Input: part model. Units: mm. Frame: model coordinates. Face numbers are marked on the shaded views. A direction names the side the tool comes from. Round coordinates to 2 decimals unless told otherwise and drop trailing zeros. Loops run counter-clockwise (first coordinate to the right, second up) from the corner with the lowest first, then second, coordinate; pieces in that order, holes last. Notation, with made-up numbers: M 20.25,-35 L 40.25,-35 A16 cw 40.25,-20 Z; hole C -10.5,-14 d11. An arc over 180 degrees is marked long. Use one line per item in the form item = value. Start each with the question number.
Q1. Ray query, line 1 along Y through (x, z) = (45, 43); line 2 along X through (y, z) = (5, 44); line 3 along Z through (x, y) = (39, 69.5). Return the intervals inside material, ascending.
Q2. Access query for the marked faces 1, 2 and 3. Directions: +Z, -Z, +X, -X, +Y, -Y. A direction counts if a zero-diameter tool reaches every point of the face in a straight line with its end or side. Return the directions, or none.
Q3. Section query D-D, the plane x = 96.5. Output: boundary loops of the cut face in (y, z), and give its area (3 significant figures).
Q4. Section query A-A, the plane x = 23.5. Output: boundary loops of the cut face in (y, z) (1 decimal), and give its area (3 significant figures).
Q5. Section query B-B, the plane y = 56. Output: boundary loops of the cut face in (x, z).
Q6. Section query C-C, the plane z = 36.5. Output: boundary loops of the cut face in (x, y).
Q7. Mould query, pull axis Y, two halves, no side actions, for the marked faces 4, 5, 6 and 7. Classes: pulls with the +Y half, pulls with the -Y half, needs draft (parallel to the pull), parting line crosses it, or undercut.
Q8. First-contact query: P1, Ø6.5, axis at x = 74.5, z = 4.5, coming from the -Y side; P2, Ø7.5, axis at y = 13.5, z = 26, coming from the +X side; P3, Ø4, axis at x = 72.5, z = 3, coming from the +Y side; P4, Ø21, axis at y = 75, z = 24, coming from the +X side. Flat tips, straight axial feed; report the tip coordinate or a pass-through.
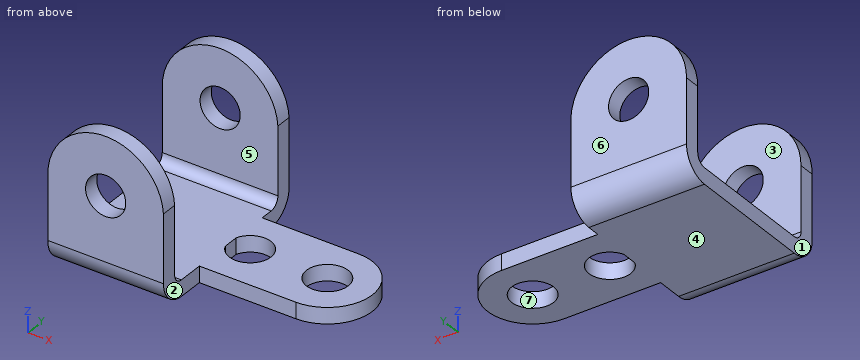
```python
from build123d import *

# Parameters (mm, degrees)
F0_R     = 10.3251
F1_DEPTH = 7.9375
F3_DEPTH = 57.0992
F4_R     = 9.92251
F5_DEPTH = 88.901
F7_DEPTH = 127.001


with BuildPart() as f1:
    # F0 (on Top) → F1 (new body)
    with BuildSketch(Plane.XY):
        with BuildLine():
            Line((0, 88.9), (0, 0))
            Line((0, 0), (50.8, 0))
            Line((50.8, 0), (50.8, 19.05))
            ThreePointArc((50.8, 19.05), (52.6598719395, 23.5401280605), (57.15, 25.4))
            Line((57.15, 25.4), (104.775, 25.4))
            ThreePointArc((104.775, 25.4), (127, 47.625), (104.775, 69.85))
            Line((104.775, 69.85), (57.15, 69.85))
            ThreePointArc((57.15, 69.85), (52.6598719395, 71.7098719395), (50.8, 76.2))
            Line((50.8, 76.2), (50.8, 88.9))
            Line((50.8, 88.9), (0, 88.9))
        make_face()
        with Locations((66.675, 47.625)):
            Circle(F0_R, mode=Mode.SUBTRACT)
        with Locations((104.775, 47.625)):
            Circle(F0_R, mode=Mode.SUBTRACT)
    extrude(amount=F1_DEPTH)

    # F2 (on Right) → F3 (join)
    with BuildSketch(Plane.YZ):
        with BuildLine():
            Line((0, 76.2), (0, 12.7))
            ThreePointArc((0, 12.7), (3.7197438789, 3.7197438789), (12.7, 0))
            Line((12.7, 0), (76.2, 0))
            ThreePointArc((76.2, 0), (85.1802561211, 3.7197438789), (88.9, 12.7))
            Line((88.9, 12.7), (88.9, 76.2))
            Line((88.9, 76.2), (80.9625, 76.2))
            Line((80.9625, 76.2), (80.9625, 12.7))
            ThreePointArc((80.9625, 12.7), (79.5675960454, 9.3324039546), (76.2, 7.9375))
            Line((76.2, 7.9375), (12.7, 7.9375))
            ThreePointArc((12.7, 7.9375), (9.3324039546, 9.3324039546), (7.9375, 12.7))
            Line((7.9375, 12.7), (7.9375, 76.2))
            Line((7.9375, 76.2), (0, 76.2))
        make_face()
    extrude(amount=F3_DEPTH)

    # F4 (on Front) → F5 (cut, through all)
    with BuildSketch(Plane.XZ):
        with Locations((28.575, 44.45)):
            Circle(F4_R)
        with BuildLine():
            Line((57.1075950167, 46.0061640709), (57.1084559489, 42.9097024275))
            ThreePointArc((57.1084559489, 42.9097024275), (57.1499988955, 44.4579449194), (57.1075950167, 46.0061640709))
        make_face()
        with BuildLine():
            ThreePointArc((0, 44.45), (27.7966291375, 73.0143967869), (57.1075950167, 46.0061640709))
            Line((57.1075950167, 46.0061640709), (57.0992, 76.2))
            Line((57.0992, 76.2), (0, 76.2))
            Line((0, 76.2), (0, 44.45))
        make_face()
    extrude(amount=-F5_DEPTH, mode=Mode.SUBTRACT)

    # F6 (on Right) → F7 (cut, through all)
    with BuildSketch(Plane.YZ):
        with BuildLine():
            Line((0, 12.7), (0, 0))
            Line((0, 0), (12.7, 0))
            ThreePointArc((12.7, 0), (3.7197438789, 3.7197438789), (0, 12.7))
        make_face()
        with BuildLine():
            Line((76.2, 0), (88.9, 0))
            Line((88.9, 0), (88.9, 12.7))
            ThreePointArc((88.9, 12.7), (85.1802561211, 3.7197438789), (76.2, 0))
        make_face()
    extrude(amount=F7_DEPTH, mode=Mode.SUBTRACT)


solid = f1.part
```
Results found:
q1.line_1 = 0 to 7.94, 80.96 to 88.9
q1.line_2 = 0 to 18.66, 38.49 to 57.1
q1.line_3 = 0 to 7.94
q2.face_1 = +Z, -Z, -X, +Y, -Y
q2.face_2 = +Z, -Z, +X, -Y
q2.face_3 = +Z, +X, -X
q3.outline = M 25.4,0 L 41.45,0 L 41.45,7.94 L 25.4,7.94 Z; M 53.8,0 L 69.85,0 L 69.85,7.94 L 53.8,7.94 Z
q3.area = 255 mm²
q4.outline = M 0,12.7 A12.7 ccw 12.7,0 L 76.2,0 A12.7 ccw 88.9,12.7 L 88.9,35.9 L 81,35.9 L 81,12.7 A4.8 cw 76.2,7.9 L 12.7,7.9 A4.8 cw 7.9,12.7 L 7.9,35.9 L 0,35.9 Z; M 0,53 L 7.9,53 L 7.9,72.6 L 0,72.6 Z; M 81,53 L 88.9,53 L 88.9,72.6 L 81,72.6 Z
q4.area = 1,400 mm²
q5.outline = M 0,0 L 60.64,0 L 60.64,7.94 L 0,7.94 Z; M 72.71,0 L 98.74,0 L 98.74,7.94 L 72.71,7.94 Z; M 110.81,0 L 125.36,0 L 125.36,7.94 L 110.81,7.94 Z
q6.outline = M 0,0 L 22.64,0 L 22.64,7.94 L 0,7.94 Z; M 0,80.96 L 22.64,80.96 L 22.64,88.9 L 0,88.9 Z; M 34.51,0 L 57.1,0 L 57.1,7.94 L 34.51,7.94 Z; M 34.51,80.96 L 57.1,80.96 L 57.1,88.9 L 34.51,88.9 Z
q7.face_4 = needs draft
q7.face_5 = undercut
q7.face_6 = pulls with the +Y half
q7.face_7 = undercut
q8.P1 = 25.4
q8.P2 = through
q8.P3 = 69.85
q8.P4 = 57.1
